Could you check a few things on this model? Use its own coordinates, in mm. Face numbers are marked on the shaded views. Round coordinates to 2 decimals unless told otherwise and drop trailing zeros. Loops run counter-clockwise (first coordinate to the right, second up) from the corner with the lowest first, then second, coordinate; pieces in that order, holes last. Notation, with made-up numbers: (-6, -21.75) - (47, -21.75) arc R15 ccw to (47, 4.25) - close; hole circle Ø2 at (65.25, 55.25). An arc over 180 degrees is marked (long way). Use one line per item in the form item = value.
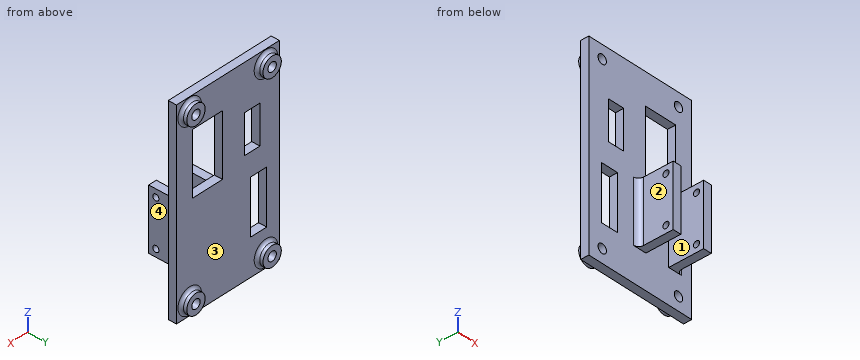
Autodesk Inventor part; units mm, degrees
ref_plane "YZ Plane" through (0, 0, 0) normal (1, 0, 0) x (0, 1, 0)
ref_plane "XZ Plane" through (0, 0, 0) normal (0, 1, 0) x (-1, 0, 0)
ref_plane "XY Plane" through (0, 0, 0) normal (0, 0, 1) x (1, 0, 0)
sketch "Sketch1" plane through (0, 0, 0) normal (0, 1, 0) x (-1, 0, 0)
  circle A0 centre (0, 0) radius 2.4
  circle A1 centre (20, 0) radius 2.4
  circle A2 centre (20, -41.5) radius 2.4
  circle A3 centre (0, -41.5) radius 2.4
  dimension "d0" = 4.8
  dimension "d4" = 20
  dimension "d5" = 41.5
extrude "Extrusion1" add sketch "Sketch1" along normal blind 1.5
sketch "Sketch2" plane through (0, 0, 0) normal (0, -1, 0) x (1, 0, 0)
  circle A0 centre (0, 0) radius 2.4 construction
  circle A1 centre (0, -41.5) radius 2.4 construction
  circle A2 centre (-20, -41.5) radius 2.4 construction
  circle A3 centre (-20, 0) radius 2.4 construction
  line L0 (3.492, 3.2394) -> (-23.508, 3.2394)
  line L1 (-23.508, 3.2394) -> (-23.508, -44.7606)
  line L2 (-23.508, -44.7606) -> (3.492, -44.7606)
  line L3 (3.492, -44.7606) -> (3.492, 3.2394)
  dimension "d8" = 27
  dimension "d9" = 48
extrude "Extrusion2" add sketch "Sketch2" along normal blind 2
sketch "Sketch3" plane through (0, -2, 0) normal (0, -1, 0) x (1, 0, 0)
  circle A0 centre (0, 0) radius 2.4 construction
  circle A1 centre (0, -41.5) radius 2.4 construction
  circle A2 centre (-20, -41.5) radius 2.4 construction
  circle A3 centre (-20, 0) radius 2.4 construction
  line L0 (-8.5471, -21.5) -> (-10.5471, -21.5)
  line L1 (-10.5471, -21.5) -> (-10.5471, -36.5)
  line L2 (-10.5471, -36.5) -> (-8.5471, -36.5)
  line L3 (-8.5471, -36.5) -> (-8.5471, -21.5)
  line L4 (-0.5471, -21.5) -> (-2.5471, -21.5)
  line L5 (-2.5471, -21.5) -> (-2.5471, -36.5)
  line L6 (-2.5471, -36.5) -> (-0.5471, -36.5)
  line L7 (-0.5471, -36.5) -> (-0.5471, -21.5)
  line L8 (0, 0) -> (0, -41.5) construction
  dimension "d12" = 2
  dimension "d13" = 2
  dimension "d14" = 15
  dimension "d15" = 6
  dimension "d17" = 5
extrude "Extrusion3" add sketch "Sketch3" along normal blind 8.5
sketch "Sketch4" plane through (-10.5471, -2, -36.5) normal (-1, 0, 0) x (0, 0, 1)
  line L0 (15, 0) -> (15, -8.5) construction
  line L1 (15, -6) -> (0, -6) construction
  line L2 (0, 0) -> (0, -8.5) construction
  circle A0 centre (13.1106, -6.75) radius 0.75
  circle A1 centre (1.8252, -6.75) radius 0.75
  line L3 (39.7394, 0) -> (-8.2606, 0)
  point P0 (36.5, 2)
  dimension "d21" = 1.5
  dimension "d22" = 0.75
  dimension "d23" = 1.5
  dimension "d24" = 0.75
  dimension "d25" = 6
extrude "Extrusion4" cut sketch "Sketch4" against normal through all
sketch "Sketch6" plane through (0, -2, 0) normal (0, -1, 0) x (1, 0, 0)
  line L0 (-0.7166, -4.3244) -> (-8.5921, -4.3244)
  line L1 (-8.5921, -4.3244) -> (-8.5921, -19.4025)
  line L2 (-8.5921, -19.4025) -> (-0.7166, -19.4025)
  line L3 (-0.7166, -19.4025) -> (-0.7166, -4.3244)
  line L4 (-14.3515, -7.8111) -> (-18.4107, -7.8111)
  line L5 (-18.4107, -7.8111) -> (-18.4107, -17.2306)
  line L6 (-18.4107, -17.2306) -> (-14.3515, -17.2306)
  line L7 (-14.3515, -17.2306) -> (-14.3515, -7.8111)
  line L8 (-15.9648, -22.747) -> (-20.1801, -22.747)
  line L9 (-20.1801, -22.747) -> (-20.1801, -35.9136)
  line L10 (-20.1801, -35.9136) -> (-15.9648, -35.9136)
  line L11 (-15.9648, -35.9136) -> (-15.9648, -22.747)
  point P0 (0, 0)
extrude "Extrusion6" cut sketch "Sketch6" against normal through all
hole "Hole1" at (0, 1.5, -41.5) direction (0, -1, 0) diameter 2.2 depth 8 tip angle 118
hole "Hole2" at (0, 1.5, 0) direction (0, -1, 0) diameter 2.2 depth 8 tip angle 118
hole "Hole3" at (-20, 1.5, -41.5) direction (0, -1, 0) diameter 2.2 depth 8 tip angle 118
hole "Hole4" at (-20, 1.5, 0) direction (0, -1, 0) diameter 2.2 depth 8 tip angle 118
fillet "Fillet1" radius 0.7 4 edges at (-17.6, 0, 0) (2.4, 0, 0) (2.4, 0, -41.5) (-17.6, 0, -41.5)
fillet "Fillet2" radius 1.3 2 edges at (-10.5471, -2, -29) (-0.5471, -2, -29)
properties part number "holder_board_basecam_simpleBCG_32bit_tiny"
1. If we section it at B-B, the plane x = -7.5: Write out the boundary of the cut face in (y, z), plus the area to 3 significant figures.
Solution:
outline = (-2, -44.76) - (0, -44.76) - (0, -19.4) - (-2, -19.4) - close; (-2, -4.32) - (0, -4.32) - (0, 3.24) - (-2, 3.24) - close
area = 65.8 mm^2
2. For P1, Ø2, axis at y = -2.5, z = -32, coming from the -X side; P2, Ø13.5, axis at x = -9, z = -15, coming from the +Y side; P3, Ø1, axis at y = -6, z = -33, coming from the -X side; P4, Ø0.9, axis at y = -8.75, z = -34.67, coming from the +X side, each with a flat end and sliding along its axis, tell me the tip position at first contact or that it passes through.
Solution:
P1 = -23.51
P2 = 0
P3 = -10.55
P4 = through
3. Please list where these lines run through material, in increasing order: line 1 along Z through (x, y) = (-20, -0.75); line 2 along Z through (x, y) = (0, -0.9); line 3 along X through (y, z) = (-4.75, -29).
Solution:
line_1 = -44.76 to -42.6, -40.4 to -35.91, -22.75 to -1.1, 1.1 to 3.24
line_2 = -44.76 to -42.6, -40.4 to -1.1, 1.1 to 3.24
line_3 = -10.55 to -8.55, -2.55 to -0.55
4. If we section it at C-C, the plane y = -8.75: Write out the boundary of the cut face in (x, z).
Solution:
outline = (-10.55, -36.5) - (-8.55, -36.5) - (-8.55, -35.42) - (-10.55, -35.42) - close; (-10.55, -33.92) - (-8.55, -33.92) - (-8.55, -24.14) - (-10.55, -24.14) - close; (-10.55, -22.64) - (-8.55, -22.64) - (-8.55, -21.5) - (-10.55, -21.5) - close; (-2.55, -36.5) - (-0.55, -36.5) - (-0.55, -35.42) - (-2.55, -35.42) - close; (-2.55, -33.92) - (-0.55, -33.92) - (-0.55, -24.14) - (-2.55, -24.14) - close; (-2.55, -22.64) - (-0.55, -22.64) - (-0.55, -21.5) - (-2.55, -21.5) - close
5. If we section it at A-A, the plane z = -41.5: Write out the boundary of the cut face in (x, y).
Solution:
outline = (-23.51, -2) - (-21.1, -2) - (-21.1, 1.5) - (-22.4, 1.5) - (-22.4, 0.7) arc R0.7 cw to (-23.1, 0) - (-23.51, 0) - close; (-18.9, -2) - (-1.1, -2) - (-1.1, 1.5) - (-2.4, 1.5) - (-2.4, 0.7) arc R0.7 cw to (-3.1, 0) - (-16.9, 0) arc R0.7 cw to (-17.6, 0.7) - (-17.6, 1.5) - (-18.9, 1.5) - close; (1.1, -2) - (3.49, -2) - (3.49, 0) - (3.1, 0) arc R0.7 cw to (2.4, 0.7) - (2.4, 1.5) - (1.1, 1.5) - close
6. If we section it at D-D, the plane y = -6.5: Write out the boundary of the cut face in (x, z), plus the area to 3 significant figures.
Solution:
outline = (-10.55, -36.5) - (-8.55, -36.5) - (-8.55, -21.5) - (-10.55, -21.5) - close; (-2.55, -36.5) - (-0.55, -36.5) - (-0.55, -21.5) - (-2.55, -21.5) - close
area = 60.0 mm^2
7. We'd pull the mould along X, two halves only. Please class the marked faces 1, 2, 3 and 4: +X half, -X half, draft (parallel to the pull), parting line (faces both ways), or undercut.
Solution:
face_1 = undercut
face_2 = -X half
face_3 = undercut
face_4 = +X half
